Input: part model. Units: mm. Frame: model coordinates. Coordinates: 2 decimals unless noted, no trailing zeros. Write each loop counter-clockwise with the first axis right and the second up, starting at its lowest first coordinate (ties: lowest second). Pieces come first, ordered by that corner, then holes. Notation, with made-up numbers: (-8.5, -1) -> (33.5, -1) arc R29 cw to (33.5, 29) -> close; hole circle Ø5 at (-30.75, -21). An arc over 180 degrees is marked (long way). Use one line per item in the form item = value. Start each with the question number.
(1) First-contact query: pin 1 (5.5 mm diameter, centred on x = -45.25, z = 64, fed in from -Y); pin 2 (6 mm diameter, centred on x = 11, z = 11, fed in from +Y). Flat tips, straight axial feed; report the tip coordinate or a pass-through.
(2) Ray query, line 1 along X through (y, z) = (4.75, 45.25); line 2 along X through (y, z) = (3.5, 64); line 3 along Z through (x, y) = (-43, 4). Return the intervals inside material, ascending.
(3) Cut plane D-D on z = -45.25. Return the cut outline in (x, y).
(4) Cut plane B-B on y = 4.25. State how many separate pieces and enclosed holes the cut face has, plus the area to 3 significant figures.
(5) Cut plane C-C on z = 64. Return the cut outline in (x, y), plus the area to 3 significant figures.
(6) Cut plane A-A on x = -45.25. Return the cut outline in (y, z), plus the area to 3 significant figures.
(7) Pull-direction query (X, two-part tool) for faces 1 (the face through (53, 3, -74)), 2 (the face through (-1, 0, -1)), 3 (the face through (-13.44, 3.13, -11.54)); classes: released by +X, released by -X, zero draft, split by the parting line, or undercut.
```python
from build123d import *

# Parameters (mm, degrees)
SKETCH2_W           = 110
SKETCH2_H           = 150
SKETCH2_R           = 3.56
SKETCH2_R_2         = 2.5
BOSS_EXTRUDE1_DEPTH = 6.35
FILLET1_R           = 5


with BuildPart() as part:
    # Sketch2 → Boss-Extrude1 (new body)
    with BuildSketch(Plane(origin=(0, 0, 0), x_dir=(1, 0, 0), z_dir=(0, 1, 0))):
        Rectangle(SKETCH2_W, SKETCH2_H)
        with Locations(Location((-45.25, 64, 0), (0, 0, 270))):
            Circle(SKETCH2_R, mode=Mode.SUBTRACT)
        with Locations(Location((-45.25, -64, 0), (0, 0, 270))):
            Circle(SKETCH2_R, mode=Mode.SUBTRACT)
        with Locations(Location((45.25, 64, 0), (0, 0, 270))):
            Circle(SKETCH2_R_2, mode=Mode.SUBTRACT)
        with Locations(Location((45.25, -64, 0), (0, 0, 270))):
            Circle(SKETCH2_R_2, mode=Mode.SUBTRACT)
        with Locations(Location((-45.25, -45.25, 0), (0, 0, 270))):
            Circle(SKETCH2_R, mode=Mode.SUBTRACT)
        with Locations(Location((45.25, -45.25, 0), (0, 0, 270))):
            Circle(SKETCH2_R, mode=Mode.SUBTRACT)
        with Locations(Location((-45.25, 45.25, 0), (0, 0, 270))):
            Circle(SKETCH2_R_2, mode=Mode.SUBTRACT)
        with Locations(Location((45.25, 45.25, 0), (0, 0, 270))):
            Circle(SKETCH2_R_2, mode=Mode.SUBTRACT)
        with Locations(Location((-11, 11, 0), (0, 0, 270))):
            Circle(SKETCH2_R_2, mode=Mode.SUBTRACT)
        with Locations(Location((11, 11, 0), (0, 0, 270))):
            Circle(SKETCH2_R_2, mode=Mode.SUBTRACT)
        with Locations(Location((11, -11, 0), (0, 0, 270))):
            Circle(SKETCH2_R_2, mode=Mode.SUBTRACT)
        with Locations(Location((-11, -11, 0), (0, 0, 270))):
            Circle(SKETCH2_R_2, mode=Mode.SUBTRACT)
    extrude(amount=BOSS_EXTRUDE1_DEPTH)

    # Fillet1
    fillet1_edges = [part.edges().sort_by_distance(p)[0] for p in [
        (-55, 3.175, -75),
        (55, 3.175, -75),
        (55, 3.175, 75),
        (-55, 3.175, 75),
    ]]
    fillet(fillet1_edges, radius=FILLET1_R)


solid = part.part
```
Values:
q1.pin_1 = through
q1.pin_2 = 6.35
q2.line_1 = -55 to -48.81, -41.69 to 41.69, 48.81 to 55
q2.line_2 = -55 to -48.81, -41.69 to 42.75, 47.75 to 55
q2.line_3 = -75 to -66.76, -61.24 to -46.34, -44.16 to 42.49, 48.01 to 61.24, 66.76 to 75
q3.outline = (-55, 0) -> (-47.75, 0) -> (-47.75, 6.35) -> (-55, 6.35) -> close; (-42.75, 0) -> (42.75, 0) -> (42.75, 6.35) -> (-42.75, 6.35) -> close; (47.75, 0) -> (55, 0) -> (55, 6.35) -> (47.75, 6.35) -> close
q4.separate_pieces = 1
q4.enclosed_holes = 12
q4.area = 16,200 mm2
q5.outline = (-55, 0) -> (-48.81, 0) -> (-48.81, 6.35) -> (-55, 6.35) -> close; (-41.69, 0) -> (42.75, 0) -> (42.75, 6.35) -> (-41.69, 6.35) -> close; (47.75, 0) -> (55, 0) -> (55, 6.35) -> (47.75, 6.35) -> close
q5.area = 622 mm2
q6.outline = (0, -75) -> (6.35, -75) -> (6.35, -67.56) -> (0, -67.56) -> close; (0, -60.44) -> (6.35, -60.44) -> (6.35, -47.75) -> (0, -47.75) -> close; (0, -42.75) -> (6.35, -42.75) -> (6.35, 41.69) -> (0, 41.69) -> close; (0, 48.81) -> (6.35, 48.81) -> (6.35, 60.44) -> (0, 60.44) -> close; (0, 67.56) -> (6.35, 67.56) -> (6.35, 75) -> (0, 75) -> close
q6.area = 785 mm2
q7.face_1 = released by +X
q7.face_2 = zero draft
q7.face_3 = undercut
